Work out the finished part from the listing and answer in its coordinate system (mm). A direction names the side the tool comes from. Coordinates: 2 decimals unless noted, no trailing zeros. Write each loop counter-clockwise with the first axis right and the second up, starting at its lowest first coordinate (ties: lowest second). Pieces come first, ordered by that corner, then holes. Notation, with made-up numbers: (18.5, 5.25) - (64.5, 5.25) arc R13 ccw to (64.5, 14.25) - close; hole circle Ø9 at (31, 65.5). An arc over 180 degrees is marked (long way). Use a Markdown table: item, result. Add a question column.
(1) Find the intervals of material crossed by line 1 (Z direction, x = 12.5, y = 13.5); line 2 (X direction, y = 0, z = -5.1); line 3 (Y direction, x = -14.5, z = -2), in increasing order. Write a range as from..to.
(2) The part is cut by section C-C, the plane y = 17.3. Give the vertices of the cut face in (x, z).
(3) The part is cut by section D-D, the plane x = 17. Give the vertices of the cut face in (y, z).
(4) The part is cut by section A-A, the plane y = 0. Give the vertices of the cut face in (x, z).
(5) For a pull along Z with two mould halves and no side action, classify faces 4 (the face through (16, -3, -7)), 5 (the face through (26, -22.5, 9)), 6 (the face through (18, 0, 0)), 7 (the face through (25.73, 15.73, 8.35)) as released by +Z, released by -Z, zero draft, split by the parting line, or undercut.
(6) A tool of negligible diameter and unlimited length cuts with its end or side. For faces 1 (the face through (27.5, 1, 4)), 2 (the face through (-9, 22.5, -2)), 3 (the face through (0, 19.5, -2)), from which of +Z, -Z, +X, -X, +Y, -Y can it reach the whole face along a straight path? Write none if from no direction.
(7) Given pin 1 Ø6 at (x, y) = (12.5, -23) entering from +Z; pin 2 Ø4 at (x, z) = (26, 11.5) entering from -Y; pin 3 Ø2.5 at (y, z) = (34.5, -1.5) entering from -X, each flat-ended and moving along its own axis, determine where each tip first touches the part or whether it passes through.
(8) The part is cut by section B-B, the plane z = 9. Give the vertices of the cut face in (x, y), then the cut area to 3 significant figures.
from build123d import *

# Parameters (mm, degrees)
SKETCH_1_W          = 55
SKETCH_1_H          = 45
EXTRUDE_1_DEPTH     = 3
SKETCH_2_W          = 3.5
SKETCH_2_H          = 45
EXTRUDE_2_DEPTH     = 12
SKETCH_3_R          = 1.7
CUT_EXTRUDE_1_DEPTH = 59.167860542
EXTRUDE_START       = -7
EXTRUDE_3_DEPTH     = 10
SKETCH_6_R          = 1.7
CUT_EXTRUDE_2_DEPTH = 66.018535195
SKETCH_7_R          = 19.2
CUT_EXTRUDE_3_DEPTH = 48.438485631
SKETCH_10_W         = 55
SKETCH_10_H         = 4
EXTRUDE_9_DEPTH     = 3


with BuildPart() as part:
    # 草图1 → 凸台-拉伸1 (new body)
    with BuildSketch(Plane.XY):
        Rectangle(SKETCH_1_W, SKETCH_1_H)
    extrude_1 = extrude(amount=EXTRUDE_1_DEPTH)

    # 草图2 → 凸台-拉伸2 (add)
    with BuildSketch(Plane.XY.offset(3)):
        with Locations((25.75, 0)):
            Rectangle(SKETCH_2_W, SKETCH_2_H)
    extrude(amount=EXTRUDE_2_DEPTH)

    # 草图3 → 切除-拉伸1 (cut, through all)
    with BuildSketch(Plane.ZY.offset(-24)):
        with Locations(Location((9, -17.3, 0), (0, 0, 270))):
            Circle(SKETCH_3_R)
        with Locations(Location((9, 17.3, 0), (0, 0, 270))):
            Circle(SKETCH_3_R)
    extrude(amount=-CUT_EXTRUDE_1_DEPTH, mode=Mode.SUBTRACT)

    # 草图5 → 凸台-拉伸3 (add)
    with BuildSketch(Plane.XY.offset(EXTRUDE_START)):
        with BuildLine():
            Line((27.5, -22.5), (9.5, -22.5))
            Line((9.5, -22.5), (21.689237996, -28.178880611))
            ThreePointArc((21.689237996, -28.178880611), (23.373199667, -29.654914404), (24, -31.804687417))
            Line((24, -31.804687417), (24, -36.744522299))
            Line((24, -36.744522299), (27.5, -36.744522299))
            Line((27.5, -36.744522299), (27.5, -22.5))
        make_face()
    extrude_3 = extrude(amount=EXTRUDE_3_DEPTH)

    # 草图6 → 切除-拉伸2 (cut, through all)
    with BuildSketch(Plane.ZY.offset(-24)):
        with Locations((0, -34.129434576)):
            Circle(SKETCH_6_R)
        with Locations((-4.607898424, -34.129434576)):
            Circle(SKETCH_6_R)
    cut_extrude_2 = extrude(amount=-CUT_EXTRUDE_2_DEPTH, mode=Mode.SUBTRACT)

    # 镜向3: 凸台-拉伸3, 切除-拉伸2 across plane
    add(extrude_3.mirror(Plane.ZX))
    add(cut_extrude_2.mirror(Plane.ZX), mode=Mode.SUBTRACT)

    # 草图7 → 切除-拉伸3 (cut, symmetric)
    with BuildSketch(Plane.XY.offset(3)):
        with Locations((-4.204977357, 0)):
            Circle(SKETCH_7_R)
    cut_extrude_3 = extrude(amount=CUT_EXTRUDE_3_DEPTH, both=True, mode=Mode.SUBTRACT)

    # 镜向6: 凸台-拉伸1, 切除-拉伸3 across plane
    add(extrude_1.mirror(Plane.XY.offset(-2)))
    add(cut_extrude_3.mirror(Plane.XY.offset(-2)), mode=Mode.SUBTRACT)

    # 草图10 → 凸台-拉伸9 (add)
    with BuildSketch(Plane(origin=(0, -22.5, 0), x_dir=(-1, 0, 0), z_dir=(0, -1, 0))):
        with Locations((0, 2)):
            Rectangle(SKETCH_10_W, SKETCH_10_H)
    extrude_9 = extrude(amount=-EXTRUDE_9_DEPTH)

    # 镜向7: 凸台-拉伸9 across plane
    add(extrude_9.mirror(Plane.ZX))


solid = part.part
Model answer:
| question | item | result |
|---|---|---|
| 1 | line 1 | -7..-4, 0..3 |
| 1 | line 2 | -27.5..-23.4, 15..27.5 |
| 1 | line 3 | -22.5..-19.5, 19.5..22.5 |
| 2 | outline | (-27.5, -7) - (-12.53, -7) - (-12.53, -4) - (-27.5, -4) - close; (-27.5, 0) - (-12.53, 0) - (-12.53, 3) - (-27.5, 3) - close; (4.12, -7) - (27.5, -7) - (27.5, -4) - (4.12, -4) - close; (4.12, 0) - (27.5, 0) - (27.5, 7.3) - (24, 7.3) - (24, 3) - (4.12, 3) - close; (24, 10.7) - (27.5, 10.7) - (27.5, 15) - (24, 15) - close |
| 3 | outline | (-25.99, -7) - (25.99, -7) - (25.99, 3) - (-25.99, 3) - close; hole (-19.5, -4) - (19.5, -4) - (19.5, 0) - (-19.5, 0) - close |
| 4 | outline | (-27.5, -7) - (-23.4, -7) - (-23.4, -4) - (-27.5, -4) - close; (-27.5, 0) - (-23.4, 0) - (-23.4, 3) - (-27.5, 3) - close; (15, -7) - (27.5, -7) - (27.5, -4) - (15, -4) - close; (15, 0) - (27.5, 0) - (27.5, 15) - (24, 15) - (24, 3) - (15, 3) - close |
| 5 | face 4 | released by -Z |
| 5 | face 5 | zero draft |
| 5 | face 6 | undercut |
| 5 | face 7 | undercut |
| 6 | face 1 | +Z, -Z, +X, +Y, -Y |
| 6 | face 2 | +Z, -Z, -X, +Y |
| 6 | face 3 | +X, -X |
| 7 | pin 1 | z = 3 |
| 7 | pin 2 | y = -22.5 |
| 7 | pin 3 | x = 24 |
| 8 | outline | (24, -22.5) - (27.5, -22.5) - (27.5, -19) - (24, -19) - close; (24, -15.6) - (27.5, -15.6) - (27.5, 15.6) - (24, 15.6) - close; (24, 19) - (27.5, 19) - (27.5, 22.5) - (24, 22.5) - close |
| 8 | area | 134 mm^2 |
